```python
from build123d import *

# Parameters (mm, degrees)
F0_R         = 3.175
F1_DEPTH     = 15.748
F2_W         = 4.953
F2_H         = 16.2648302115
F2_H_2       = 7.994236929
F3_DEPTH     = 12.7
F2_W_2       = 2.032
F2_H_3       = 20.5828301237
F4_DEPTH     = 12.7
F5_T4_DEPTH  = 29.7595972634
F5_T10_DEPTH = 29.7595972634
F7_D         = 2.5273


# Not quite as in the source:
# - a fillet or chamfer that OpenCascade refuses, or shapes differently, is made with other operations: its cross-section is extruded or revolved along the edge and cut away or added


with BuildPart() as f1:
    # F0 (on Front) → F1 (new body)
    with BuildSketch(Plane.XZ):
        with BuildLine():
            Line((-8.89, 21.8948), (-6.3090456189, -0.7200301237))
            ThreePointArc((-6.3090456189, -0.7200301237), (0, -6.35), (6.3090456189, -0.7200301237))
            Line((6.3090456189, -0.7200301237), (8.89, 21.8948))
            Line((8.89, 21.8948), (-8.89, 21.8948))
        make_face()
        Circle(F0_R, mode=Mode.SUBTRACT)
    extrude(amount=F1_DEPTH)

    # F2 (on Right) → F3 (cut, symmetric)
    with BuildSketch(Plane.YZ):
        with Locations((-7.874, 7.4123849821)):
            Rectangle(F2_W, F2_H)
        with Locations((-7.874, -4.7171485882)):
            Rectangle(F2_W, F2_H_2)
    extrude(amount=F3_DEPTH, both=True, mode=Mode.SUBTRACT)

    # F2 (on Right) → F4 (cut, symmetric)
    with BuildSketch(Plane.YZ):
        with Locations((-14.732, -4.7171485882)):
            Rectangle(F2_W_2, F2_H_2)
        with Locations((-1.016, -4.7171485882)):
            Rectangle(F2_W_2, F2_H_2)
        with Locations((-1.016, 9.5713849382)):
            Rectangle(F2_W_2, F2_H_3)
        with Locations((-14.732, 9.5713849382)):
            Rectangle(F2_W_2, F2_H_3)
    extrude(amount=F4_DEPTH, both=True, mode=Mode.SUBTRACT)

    # F5: fillet of radius 2.54 on 2 edges, made by hand


with BuildPart() as f5_tool2:
    # F5_s3 → F5_t4 (new body)
    with BuildSketch(Plane.YZ.offset(-14.8797986317)):
        with BuildLine():
            ThreePointArc((-15.748, 19.8628), (-14.2885244601, 18.9805554727), (-13.716, 17.3741184213))
            Line((-13.716, 17.3741184213), (-13.716, 19.8628))
            Line((-13.716, 19.8628), (-15.748, 19.8628))
        make_face()
    extrude(amount=F5_T4_DEPTH)

    split(bisect_by=Plane(origin=(6.3090456189, 0, -0.7200301237), x_dir=(0, 1, 0), z_dir=(-0.9935504912, 0, 0.1133905707)), keep=Keep.TOP)

    split(bisect_by=Plane(origin=(-6.3090456189, 0, -0.7200301237), x_dir=(0, 1, 0), z_dir=(0.9935504912, 0, 0.1133905707)), keep=Keep.TOP)


with BuildPart() as f1_1:
    add(f1.part)

    # F5_t1: union F5_tool2
    add(f5_tool2.part)


with BuildPart() as f5_tool8:
    # F5_s9 → F5_t10 (new body)
    with BuildSketch(Plane.YZ.offset(14.8797986317)):
        with BuildLine():
            ThreePointArc((-2.032, 17.3741184213), (-1.4594755399, 18.9805554727), (0, 19.8628))
            Line((0, 19.8628), (-2.032, 19.8628))
            Line((-2.032, 19.8628), (-2.032, 17.3741184213))
        make_face()
    extrude(amount=-F5_T10_DEPTH)

    split(bisect_by=Plane(origin=(6.3090456189, 0, -0.7200301237), x_dir=(0, 1, 0), z_dir=(-0.9935504912, 0, 0.1133905707)), keep=Keep.TOP)

    split(bisect_by=Plane(origin=(-6.3090456189, 0, -0.7200301237), x_dir=(0, 1, 0), z_dir=(0.9935504912, 0, 0.1133905707)), keep=Keep.TOP)


with BuildPart() as f1_2:
    add(f1_1.part)

    # F5_t7: union F5_tool8
    add(f5_tool8.part)

    # F7 (through all)
    with Locations(Plane.XY.offset(21.8948)):
        with Locations((-5.842, -7.874), (5.842, -7.874)):
            Hole(F7_D / 2)


solid = f1_2.part
```
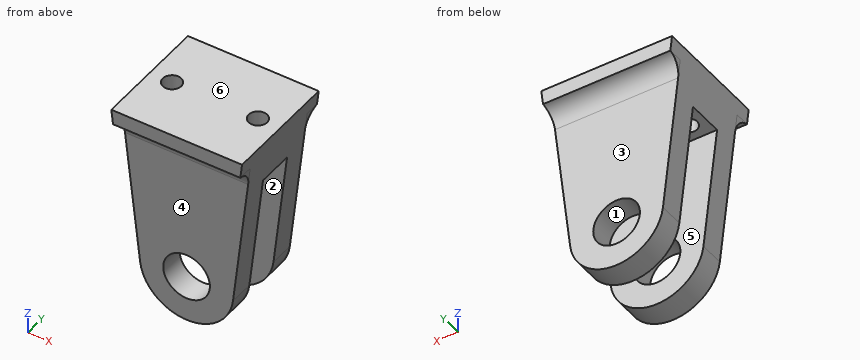
Geometry: final body of the model. Coordinates: model frame, mm. Face numbers are marked on the shaded views. A direction names the side the tool comes from. Coordinates: 2 decimals unless noted, no trailing zeros. Order: outer loops, then holes, each group sorted by start corner. A loop starts at its lowest first (then second) coordinate and runs counter-clockwise, first axis right, second up. Notation, with made-up numbers: (40, 47) -> (67, 47) arc R13 ccw to (67, 57) -> close; hole circle Ø1 at (48, -20). An arc over 180 degrees is marked (long way). Answer in a Markdown table with one row per item.
Item 1: Section A-A on x = 0. State how many separate pieces and enclosed holes the cut face has, plus the area to 3 significant figures.
Return value:
| item | result |
|---|---|
| separate pieces | 3 |
| enclosed holes | 0 |
| area | 190 mm² |
Item 2: Section D-D on z = 0. Output: boundary loops of the cut face in (x, y) (1 decimal), plus the area to 3 significant figures.
Return value:
| item | result |
|---|---|
| outline | (-6.4, -13.7) -> (-3.2, -13.7) -> (-3.2, -10.4) -> (-6.4, -10.4) -> close; (-6.4, -5.4) -> (-3.2, -5.4) -> (-3.2, -2) -> (-6.4, -2) -> close; (3.2, -13.7) -> (6.4, -13.7) -> (6.4, -10.4) -> (3.2, -10.4) -> close; (3.2, -5.4) -> (6.4, -5.4) -> (6.4, -2) -> (3.2, -2) -> close |
| area | 43.3 mm² |
Item 3: Section B-B on z = 14.25. Output: boundary loops of the cut face in (x, y), plus the area to 3 significant figures.
Return value:
| item | result |
|---|---|
| outline | (-8.02, -13.72) -> (8.02, -13.72) -> (8.02, -10.35) -> (-8.02, -10.35) -> close; (-8.02, -5.4) -> (8.02, -5.4) -> (8.02, -2.03) -> (-8.02, -2.03) -> close |
| area | 108 mm² |
Item 4: Contact query for flat-ended pins moving along their axis: P1, Ø5, axis at x = 1.5, z = 9, coming from the -Y side; P2, Ø8, axis at y = -14, z = 15, coming from the +X side; P3, Ø2, axis at x = -0.5, z = 12, coming from the +Y side. Output: stop coordinate, or through.
Return value:
| item | result |
|---|---|
| P1 | stops at y = -13.72 |
| P2 | stops at x = 8.56 |
| P3 | stops at y = -2.03 |
Item 5: Ray query, L1, parallel to Y at x = -5.75, z = 11.75; L2, parallel to X at y = -3.9, z = 0 (3 decimals); L3, parallel to Y at x = 4.25, z = 17.5. Return the intervals inside material, ascending.
Return value:
| item | result |
|---|---|
| L1 | y = -13.72 to -10.35, -5.4 to -2.03 |
| L2 | x = -6.391 to -3.175, 3.175 to 6.391 |
| L3 | y = -13.72 to -2.03 |
Item 6: Section C-C on y = -8.25. Output: boundary loops of the cut face in (x, z).
Return value:
| item | result |
|---|---|
| outline | (-8.89, 21.89) -> (-8.17, 15.54) -> (-7.05, 15.54) -> (-7.05, 21.89) -> close; (-4.64, 15.54) -> (4.64, 15.54) -> (4.64, 21.89) -> (-4.64, 21.89) -> close; (7.05, 15.54) -> (8.17, 15.54) -> (8.89, 21.89) -> (7.05, 21.89) -> close |
Item 7: Access query for the marked faces 4, 5 and 6. Directions: +Z, -Z, +X, -X, +Y, -Y. A direction counts if a zero-diameter tool reaches every point of the face in a straight line with its end or side. Return the directions, or none.
Return value:
| item | result |
|---|---|
| face 4 | -Z, +X, -X, -Y |
| face 5 | -Z, +X, -X |
| face 6 | +Z, +X, -X, +Y, -Y |
Item 8: Draft query along Y for the marked faces 1, 2 and 3. Return one class per face: released by +Y, released by -Y, zero draft, split by the parting line, or undercut.
Return value:
| item | result |
|---|---|
| face 1 | zero draft |
| face 2 | undercut |
| face 3 | released by +Y |
